Model file for the job. Use its own axes, mm. Give positions to 0.01 mm unless a question says otherwise; leave off trailing zeros. Write each loop counter-clockwise with the first axis right and the second up, starting at its lowest first coordinate (ties: lowest second). Pieces come first, ordered by that corner, then holes. Notation, with made-up numbers: (-0.5, 72) - (58.5, 72) arc R27 cw to (58.5, 91) - close; hole circle Ø3 at (34, -33.75). An arc over 180 degrees is marked (long way). One line per item, written item: value. Start each with the question number.
(1) Drop a flat-ended pin along its axis: P1, Ø2, axis at x = -34, y = -4.5, coming from the -Z side. Give the stop position or say it passes through.
(2) Mould opens along Y. For faces 1 (the face through (-25, 3, 0)), 2 (the face through (-25, -9.892, 3)), 3 (the face through (-3.45, 1.6, 3.22)) say: pulls with the +Y half, pulls with the -Y half, needs draft (parallel to the pull), parting line crosses it, or undercut.
(3) Probe L1, parallel to X at y = 2.75, z = 0.75; L2, parallel to X at y = 1.5, z = 1. List the from-to ranges inside material, lowest first.
(4) Cut at B-B, the plane x = -3. List the corners of the cut face in (y, z).
(5) Cut at A-A, the plane y = 3.5. List the corners of the cut face in (x, z).
Autodesk Inventor part; units mm, degrees
ref_plane "YZ Plane" through (0, 0, 0) normal (1, 0, 0) x (0, 1, 0)
ref_plane "XZ Plane" through (0, 0, 0) normal (0, 1, 0) x (-1, 0, 0)
ref_plane "XY Plane" through (0, 0, 0) normal (0, 0, 1) x (1, 0, 0)
sketch "Sketch1" plane through (0, 0, 0) normal (0, 0, 1) x (1, 0, 0)
  line L0 (-53.9057, 15.5084) -> (-1.8807, 15.5084)
  line L1 (-1.8807, 15.5084) -> (-1.8807, -9.8916)
  line L2 (-1.8807, -9.8916) -> (-53.9057, -9.8916)
  line L3 (-53.9057, -9.8916) -> (-53.9057, 15.5084)
  point P0 (0, 0)
  dimension "d0" = 52.025
  dimension "d1" = 25.4
extrude "Extrusion1" add sketch "Sketch1" along normal blind 6.35
sketch "Sketch2" plane through (-1.8807, -9.8916, 0) normal (1, 0, 0) x (0, 0, -1)
  line L0 (-6.35, 25.4) -> (-6.35, 0)
  line L1 (0, 0) -> (-6.35, 0)
  line L2 (0, 25.4) -> (0, 0)
  line L3 (0, 25.4) -> (-6.35, 25.4)
  point P0 (0, 9.8916)
extrude "Extrusion2" add sketch "Sketch2" along normal blind 12.7
sketch "Sketch3" plane through (0, 0, 6.35) normal (0, 0, 1) x (1, 0, 0)
  line L0 (10.8193, -9.8916) -> (10.8193, 15.5084)
  line L1 (10.8193, -9.8916) -> (10.8193, 2.8084)
  line L2 (10.8193, 2.8084) -> (-1.8807, 2.8084)
  circle A0 centre (-1.8807, 2.8084) radius 1.9812
  point P0 (0, 0)
  dimension "d6" = 12.7
  dimension "d7" = 3.9624
extrude "Extrusion3" cut sketch "Sketch3" against normal blind 12.7
sketch "Sketch4" plane through (-53.9057, -9.8916, 0) normal (-1, 0, 0) x (0, 0, 1)
  line L0 (6.35, 0) -> (6.35, 25.4)
  line L1 (0, 25.4) -> (6.35, 25.4)
  line L2 (0, 0) -> (0, 25.4)
  line L3 (0, 0) -> (6.35, 0)
  point P0 (0, 9.8916)
extrude "Extrusion4" add sketch "Sketch4" along normal blind 6.35
sketch "Sketch5" plane through (-60.2557, -9.8916, 0) normal (-1, 0, 0) x (0, 0, 1)
  line L0 (6.35, 0) -> (0, 0)
  line L1 (6.35, 25.4) -> (6.35, 0)
  line L2 (0, 25.4) -> (6.35, 25.4)
  line L3 (0, 0) -> (0, 25.4)
  point P0 (0, 9.8916)
extrude "Extrusion5" add sketch "Sketch5" along normal blind 1.1684
properties part number "hconnector2"
Answers follow:
1. P1: stops at z = 0
2. face 1: needs draft
2. face 2: pulls with the -Y half
2. face 3: undercut
3. L1: x = -61.42 to -3.86, 0.1 to 10.82
3. L2: x = -61.42 to -3.37, -0.39 to 10.82
4. outline: (-9.89, 0) - (1.17, 0) - (1.17, 6.35) - (-9.89, 6.35) - close; (4.44, 0) - (15.51, 0) - (15.51, 6.35) - (4.44, 6.35) - close
5. outline: (-61.42, 0) - (-3.74, 0) - (-3.74, 6.35) - (-61.42, 6.35) - close; (-0.02, 0) - (10.82, 0) - (10.82, 6.35) - (-0.02, 6.35) - close
